from build123d import *

# Parameters (mm, degrees)
SKETCH1_R                    = 12.7
BOSS_EXTRUDE1_DEPTH          = 12.7
SKETCH2_R                    = 25.4
BOSS_EXTRUDE2_DEPTH          = 6.35
SKETCH3_R                    = 3.3734375
CUT_EXTRUDE1_DEPTH           = 20.05
H_0_266_DIAMETER_HOLE1_D     = 6.7564
H_0_266_DIAMETER_HOLE1_DEPTH = 25.4
H_0_266_DIAMETER_HOLE1_TIP   = 2.029827343


with BuildPart() as part:
    # Sketch1 → Boss-Extrude1 (new body)
    with BuildSketch(Plane(origin=(0, 0, 0), x_dir=(1, 0, 0), z_dir=(0, 1, 0))):
        Circle(SKETCH1_R)
    extrude(amount=BOSS_EXTRUDE1_DEPTH)

    # Sketch2 → Boss-Extrude2 (add)
    with BuildSketch(Plane(origin=(0, 12.7, 0), x_dir=(1, 0, 0), z_dir=(0, 1, 0))):
        Circle(SKETCH2_R)
    extrude(amount=BOSS_EXTRUDE2_DEPTH)

    # Sketch3 → Cut-Extrude1 (cut, through all)
    with BuildSketch(Plane(origin=(0, 19.05, 0), x_dir=(1, 0, 0), z_dir=(0, 1, 0))):
        Circle(SKETCH3_R)
    extrude(amount=-CUT_EXTRUDE1_DEPTH, mode=Mode.SUBTRACT)

    # H (0.266) Diameter Hole1
    with Locations(Plane(origin=(0, 19.05, 0), x_dir=(1, 0, 0), z_dir=(0, 1, 0))):
        with Locations((0, 19.05), (-16.497783942, -9.525), (16.497783942, -9.525)):
            Hole(H_0_266_DIAMETER_HOLE1_D / 2, depth=H_0_266_DIAMETER_HOLE1_DEPTH)
            with Locations((0, 0, -(H_0_266_DIAMETER_HOLE1_DEPTH + H_0_266_DIAMETER_HOLE1_TIP / 2))):  # 118° drill point
                Cone(0, H_0_266_DIAMETER_HOLE1_D / 2, H_0_266_DIAMETER_HOLE1_TIP, mode=Mode.SUBTRACT)

    # Sketch8 → #10 (0.1935) Diameter Hole1 (revolve, cut)
    with BuildSketch(Plane(origin=(0, 6.35, 0), x_dir=(0, 1, 0), z_dir=(1, 0, 0))):
        Polygon((0, 0), (0, 26.876584928), (2.45745, 25.4), (2.45745, 0), align=None)
    revolve(axis=Axis((0, 6.35, -6.35), (0, 0, 1)), mode=Mode.SUBTRACT)


solid = part.part
Verification items for the finished model (mm, model axes). A direction names the side the tool comes from. Coordinates: 2 decimals unless noted, no trailing zeros. Order: outer loops, then holes, each group sorted by start corner. A loop starts at its lowest first (then second) coordinate and runs counter-clockwise, first axis right, second up.
1. Go/stop test with flat-tipped pins: pin 1 Ø6 at (y, z) = (7, 0) entering from +X; pin 2 Ø8 at (x, y) = (5, 16) entering from +Z; pin 3 Ø6 at (x, z) = (0, -19.05) entering from -Y; pin 4 Ø8 at (x, z) = (16.5, 9.52) entering from -Y. Record where each tip stops, or that it passes through.
Results found:
pin 1: stops at x = 12.7
pin 2: stops at z = 25.38
pin 3: passes through
pin 4: stops at y = 12.7
2. Sectioned sample at B-B, the plane x = 0. Record the cut outline in (y, z).
Results found:
outline: (0, -12.7) - (12.7, -12.7) - (12.7, -15.67) - (19.05, -15.67) - (19.05, -3.37) - (0, -3.37) - close; (0, 3.37) - (3.89, 3.37) - (3.89, 12.7) - (0, 12.7) - close; (8.81, 3.37) - (19.05, 3.37) - (19.05, 25.4) - (12.7, 25.4) - (12.7, 12.7) - (8.81, 12.7) - close; (12.7, -25.4) - (19.05, -25.4) - (19.05, -22.43) - (12.7, -22.43) - close
3. Sectioned sample at C-C, the plane x = -18. Record the cut outline in (y, z), and give its area (3 significant figures).
Results found:
outline: (12.7, -17.92) - (19.05, -17.92) - (19.05, 6.5) - (12.7, 6.5) - close; (12.7, 12.55) - (19.05, 12.55) - (19.05, 17.92) - (12.7, 17.92) - close
area: 189 mm2
4. Release check for a two-part mould opening along Z. For faces 3 (the face through (0.73, 15.83, -15.75)), 4 (the face through (-5.506, 15.831, 24.796)), 5 (the face through (0.94, 8.62, 7.44)), 6 (the face through (19.18, 15.83, 11.58)) record: +Z half, -Z half, draft (parallel to the pull), parting line (faces both ways), or undercut.
Results found:
face 3: undercut
face 4: parting line
face 5: draft
face 6: undercut
5. Sectioned sample at D-D, the plane z = -19.05. Record the cut outline in (x, y), and give its area (3 significant figures).
Results found:
outline: (-16.8, 12.7) - (-3.38, 12.7) - (-3.38, 19.05) - (-16.8, 19.05) - close; (3.38, 12.7) - (16.8, 12.7) - (16.8, 19.05) - (3.38, 19.05) - close
area: 170 mm2
6. Scan lines: line 1 (Z direction, x = 0, y = 11); line 2 (Y direction, x = -2.5, z = 16); line 3 (X direction, y = 16.5, z = -19.05). Record each from-to range of solid material in increasing order.
Results found:
line 1: z = -12.7 to -3.37, 3.37 to 12.7
line 2: y = 12.7 to 19.05
line 3: x = -16.8 to -3.38, 3.38 to 16.8
7. Set-up check for faces 1 (the face through (-18.1, 15.8, 12.5)), 2 (the face through (-2.75, 6.26, 12.4)): record each of +Z, -Z, +X, -X, +Y, -Y from which the full face is reachable in a straight line by a thin tool's end or side.
Results found:
face 1: +Y, -Y
face 2: -Y
8. Sectioned sample at A-A, the plane z = 0. Record the cut outline in (x, y).
Results found:
outline: (-25.4, 12.7) - (-12.7, 12.7) - (-12.7, 0) - (-3.37, 0) - (-3.37, 19.05) - (-25.4, 19.05) - close; (3.37, 0) - (12.7, 0) - (12.7, 12.7) - (25.4, 12.7) - (25.4, 19.05) - (3.37, 19.05) - close
